from build123d import *

# Parameters (mm, degrees)
SKETCH1_W                    = 30
SKETCH1_H                    = 15
BASE_FLANGE1_DEPTH           = 3.175
EDGE_FLANGE1_STRIP_W         = 18.7
EDGE_FLANGE1_STRIP_H         = 3.175
EDGE_FLANGE1_STRIP_CUT_DEPTH = 15
EDGE_FLANGE1_DEPTH           = 15
EDGE_FLANGE2_STRIP_W         = 18.7
EDGE_FLANGE2_STRIP_H         = 3.175
EDGE_FLANGE2_STRIP_CUT_DEPTH = 15
EDGE_FLANGE2_DEPTH           = 15
SKETCH14_R                   = 5.08
CUT_EXTRUDE1_DEPTH           = 82.072299394
SKETCH15_R                   = 2.54
CUT_EXTRUDE2_DEPTH           = 10
FILLET1_R                    = 3


# Sheet-metal steps are written as plain solids
with BuildPart() as part:
    # Sketch1 → Base-Flange1 (new body)
    with BuildSketch(Plane.XY):
        Rectangle(SKETCH1_W, SKETCH1_H)
    extrude(amount=-BASE_FLANGE1_DEPTH)

    # Edge-Flange1 strip (across the edge) → Edge-Flange1 strip cut (cut)
    with BuildSketch(Plane(origin=(15, -7.5, 0), x_dir=(-1, 0, 0), z_dir=(0, 1, 0))):
        with Locations((-6.35, -1.5875)):
            Rectangle(EDGE_FLANGE1_STRIP_W, EDGE_FLANGE1_STRIP_H)
    extrude(amount=EDGE_FLANGE1_STRIP_CUT_DEPTH, mode=Mode.SUBTRACT)

    # Edge-Flange1 section (across the edge) → Edge-Flange1 (add)
    with BuildSketch(Plane(origin=(15, -7.5, 0), x_dir=(-1, 0, 0), z_dir=(0, 1, 0))):
        with BuildLine():
            Line((-3.175, 3), (-3.175, 75.477))
            Line((-3.175, 75.477), (0, 75.477))
            Line((0, 75.477), (0, 3))
            ThreePointArc((0, 3), (0.878679656, 0.878679656), (3, 0))
            Line((3, 0), (3, -3.175))
            ThreePointArc((3, -3.175), (-1.366384374, -1.366384374), (-3.175, 3))
        make_face()
    extrude(amount=EDGE_FLANGE1_DEPTH)

    # Edge-Flange2 strip (across the edge) → Edge-Flange2 strip cut (cut)
    with BuildSketch(Plane(origin=(15, -7.5, 75.477), x_dir=(0, 0, -1), z_dir=(0, 1, 0))):
        with Locations((-6.35, -1.5875)):
            Rectangle(EDGE_FLANGE2_STRIP_W, EDGE_FLANGE2_STRIP_H)
    extrude(amount=EDGE_FLANGE2_STRIP_CUT_DEPTH, mode=Mode.SUBTRACT)

    # Edge-Flange2 section (across the edge) → Edge-Flange2 (add)
    with BuildSketch(Plane(origin=(15, -7.5, 75.477), x_dir=(0, 0, -1), z_dir=(0, 1, 0))):
        with BuildLine():
            Line((-3.175, 3), (-3.175, 25.195))
            Line((-3.175, 25.195), (0, 25.195))
            Line((0, 25.195), (0, 3))
            ThreePointArc((0, 3), (0.878679656, 0.878679656), (3, 0))
            Line((3, 0), (3, -3.175))
            ThreePointArc((3, -3.175), (-1.366384374, -1.366384374), (-3.175, 3))
        make_face()
    extrude(amount=EDGE_FLANGE2_DEPTH)

    # Sketch14 → Cut-Extrude1 (cut, through all)
    with BuildSketch(Plane.XY):
        with Locations((-7.38, 0)):
            Circle(SKETCH14_R)
    extrude(amount=-CUT_EXTRUDE1_DEPTH, mode=Mode.SUBTRACT)

    # Sketch15 → Cut-Extrude2 (cut)
    with BuildSketch(Plane.XY.offset(78.652)):
        with Locations((-5.115, 0)):
            Circle(SKETCH15_R)
    extrude(amount=-CUT_EXTRUDE2_DEPTH, mode=Mode.SUBTRACT)

    # Fillet1
    fillet1_edges = [part.edges().sort_by_distance(p)[0] for p in [
        (-10.195, -7.5, 77.0645),
        (-10.195, 7.5, 77.0645),
        (-15, -7.5, -1.5875),
        (-15, 7.5, -1.5875),
    ]]
    fillet(fillet1_edges, radius=FILLET1_R)


solid = part.part
Design review of the part built by this model. Coordinates are the model's own, in mm. A direction names the side the tool comes from. Coordinates: 2 decimals unless noted, no trailing zeros. Loops run counter-clockwise (first coordinate to the right, second up) from the corner with the lowest first, then second, coordinate; pieces in that order, holes last. Notation, with made-up numbers: (62, 38) - (96, 38) arc R22 cw to (96, 46) - close; hole circle Ø7 at (-25, -30.5). An arc over 180 degrees is marked (long way). Use CSV: the item, a comma, the result in double quotes. Start each with the question number.
1. To check wall thickness, follow probe 1 along Z at (x, y) = (2, 0.75) (3 decimals); probe 2 along Y at (x, z) = (-7, -1); probe 3 along Z at (x, y) = (-11.5, -3.5) (3 decimals). State the ranges of each line that lie inside material, in increasing order.
2. Add section C-C on x = -5.5. Give the boundary of the cut face in (y, z) (3 decimals), plus the area to 3 significant figures.
3. Add section B-B on x = 4. Give the boundary of the cut face in (y, z) (3 decimals), plus the area to 4 significant figures.
4. Mouldability with a two-part tool opening along X and no side actions: class faces 1 (the flat face through (-2, 0, 0)), 2 (the cylindrical face through (-7.131, -1.546, 77.087)), 3 (the cylindrical face through (-14.1, 6.64, -1.61)) as released by +X, released by -X, zero draft, split by the parting line, or undercut.
5. For faces 4 (the cylindrical face through (-9.293, 6.645, 77.042)), 5 (the cylindrical face through (-11.124, 3.433, -1.565)), 6 (the cylindrical face through (-9.293, -6.645, 77.042)), list the 3-axis set-ups (+Z, -Z, +X, -X, +Y, -Y) from which the entire face can be reached by the end or side of a thin tool; tool diameter is ignored.
6. Add section A-A on y = 0. Give the boundary of the cut face in (x, z) (3 decimals).
7. Add section D-D on z = 12.5. Give the boundary of the cut face in (x, y) (3 decimals).
8. Clearance check with flat-ended pins moving along their axes: pin 1 (5 mm diameter, centred on y = -6, z = 61.5, fed in from -X); pin 2 (3.5 mm diameter, centred on y = 0, z = 77, fed in from -X) (3 decimals); pin 3 (5 mm diameter, centred on x = 12.5, y = 5, fed in from -Z) (3 decimals). State where each tip first meets the part, or that it passes through.
Resolved:
1,probe 1,"-3.175 to 0, 75.477 to 78.652"
1,probe 2,"-7.5 to -5.07, 5.07 to 7.5"
1,probe 3,"-3.175 to 0"
2,outline,"(-7.5, -3.175) - (-4.719, -3.175) - (-4.719, 0) - (-7.5, 0) - close; (-7.5, 75.477) - (-2.511, 75.477) - (-2.511, 78.652) - (-7.5, 78.652) - close; (2.511, 75.477) - (7.5, 75.477) - (7.5, 78.652) - (2.511, 78.652) - close; (4.719, -3.175) - (7.5, -3.175) - (7.5, 0) - (4.719, 0) - close"
2,area,"49.3 mm2"
3,outline,"(-7.5, -3.175) - (7.5, -3.175) - (7.5, 0) - (-7.5, 0) - close; (-7.5, 75.477) - (7.5, 75.477) - (7.5, 78.652) - (-7.5, 78.652) - close"
3,area,"95.25 mm2"
4,face 1,"zero draft"
4,face 2,"undercut"
4,face 3,"released by -X"
5,face 4,"+Z, -X, +Y"
5,face 5,"-Z"
5,face 6,"+Z, -X, -Y"
6,outline,"(-15, -3.175) - (-12.46, -3.175) - (-12.46, 0) - (-15, 0) - close; (-10.195, 75.477) - (-7.655, 75.477) - (-7.655, 78.652) - (-10.195, 78.652) - close; (-2.575, 75.477) - (12, 75.477) arc R3 cw to (15, 72.477) - (15, 3) arc R3 cw to (12, 0) - (-2.3, 0) - (-2.3, -3.175) - (12, -3.175) arc R6.175 ccw to (18.175, 3) - (18.175, 72.477) arc R6.175 ccw to (12, 78.652) - (-2.575, 78.652) - close"
7,outline,"(15, -7.5) - (18.175, -7.5) - (18.175, 7.5) - (15, 7.5) - close"
8,pin 1,"x = 15"
8,pin 2,"x = -10.195"
8,pin 3,"z = -3.175"
